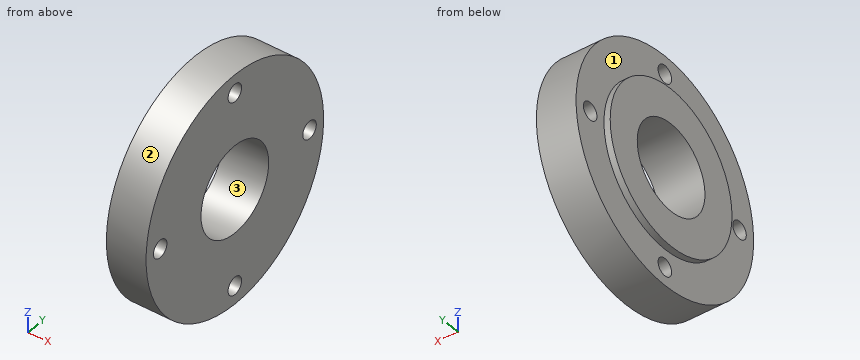
```python
from build123d import *

# Parameters (mm, degrees)
SKETCH1_R             = 32.766
BOSS_EXTRUDE1_DEPTH   = 11.303
SKETCH2_R             = 22.479
BOSS_EXTRUDE2_DEPTH   = 1.778
SKETCH3_R             = 12.5
CUT_EXTRUDE1_DEPTH    = 49.149081746
M6_TAPPED_HOLE1_D     = 5
M6_TAPPED_HOLE1_DEPTH = 12.446
M6_TAPPED_HOLE1_TIP   = 1.502151548


with BuildPart() as part:
    # Sketch1 → Boss-Extrude1 (new body)
    with BuildSketch(Plane(origin=(0, 0, 0), x_dir=(0, 0, -1), z_dir=(1, 0, 0))):
        Circle(SKETCH1_R)
    extrude(amount=-BOSS_EXTRUDE1_DEPTH)

    # Sketch2 → Boss-Extrude2 (add)
    with BuildSketch(Plane.ZY.offset(11.303)):
        with Locations(Location((0, 0, 0), (0, 0, 180))):
            Circle(SKETCH2_R)
    extrude(amount=BOSS_EXTRUDE2_DEPTH)

    # Sketch3 → Cut-Extrude1 (cut, through all)
    with BuildSketch(Plane.ZY.offset(13.081)):
        Circle(SKETCH3_R)
    extrude(amount=-CUT_EXTRUDE1_DEPTH, mode=Mode.SUBTRACT)

    # M6 Tapped Hole1
    with Locations(Plane.ZY.offset(11.303)):
        with Locations((0, 27.559), (27.559, 0), (0, -27.559), (-27.559, 0)):
            Hole(M6_TAPPED_HOLE1_D / 2, depth=M6_TAPPED_HOLE1_DEPTH)
            with Locations((0, 0, -(M6_TAPPED_HOLE1_DEPTH + M6_TAPPED_HOLE1_TIP / 2))):  # 118° drill point
                Cone(0, M6_TAPPED_HOLE1_D / 2, M6_TAPPED_HOLE1_TIP, mode=Mode.SUBTRACT)


solid = part.part
```
For this review, take the finished solid that the model builds, in its own axes (mm). Face numbers are marked on the shaded views. Coordinates: 2 decimals unless noted, no trailing zeros. Loops run counter-clockwise (first coordinate to the right, second up) from the corner with the lowest first, then second, coordinate; pieces in that order, holes last.
1. For line 1 (Y direction, x = -5.25, z = 0); line 2 (Y direction, x = -12.5, z = 0.5); line 3 (Y direction, x = -7.25, z = 1.5), list the stretches that pass through material, from the lowest coordinate up.
2. Insertion check: P1, Ø2, axis at x = -9.5, z = 16, coming from the -Y side; P2, Ø1, axis at x = -10, z = 4, coming from the -Y side; P3, Ø12, axis at y = -14.5, z = 25.5, coming from the -X side; P4, Ø12, axis at y = 5.5, z = 15.5, coming from the +X side. Each pin has a flat end and moves straight along its axis. Give the tip position at first contact, or say it passes through.
3. Add section A-A, the plane y = 0. Give the boundary of the cut face in (x, z), then the cut area to 3 significant figures.
4. Mouldability with a two-part tool opening along Z and no side actions: class the marked faces 1, 2 and 3 as +Z half, -Z half, draft (parallel to the pull), parting line (faces both ways), or undercut.
5. Add section C-C, the plane y = -7.5. Give the boundary of the cut face in (x, z), then the cut area to 3 significant figures.
6. Add section D-D, the plane z = -28.5. Give the boundary of the cut face in (x, y), then the cut area to 3 significant figures.
Result:
1. line 1: y = -32.77 to -30.06, -25.06 to -12.5, 12.5 to 25.06, 30.06 to 32.77
1. line 2: y = -22.47 to -12.49, 12.49 to 22.47
1. line 3: y = -32.73 to -29.56, -25.56 to -12.41, 12.41 to 25.56, 29.56 to 32.73
2. P1: stops at y = -29.13
2. P2: stops at y = -32.58
2. P3: stops at x = -11.3
2. P4: stops at x = 0
3. outline: (-13.08, -22.48) - (-11.3, -22.48) - (-11.3, -25.06) - (0, -25.06) - (0, -12.5) - (-13.08, -12.5) - close; (-13.08, 12.5) - (0, 12.5) - (0, 25.06) - (-11.3, 25.06) - (-11.3, 22.48) - (-13.08, 22.48) - close; (-11.3, -32.77) - (0, -32.77) - (0, -30.06) - (-11.3, -30.06) - close; (-11.3, 30.06) - (0, 30.06) - (0, 32.77) - (-11.3, 32.77) - close
3. area: 381 mm2
4. face 1: draft
4. face 2: parting line
4. face 3: undercut
5. outline: (-13.08, -21.19) - (-11.3, -21.19) - (-11.3, -31.9) - (0, -31.9) - (0, -10) - (-13.08, -10) - close; (-13.08, 10) - (0, 10) - (0, 31.9) - (-11.3, 31.9) - (-11.3, 21.19) - (-13.08, 21.19) - close
5. area: 535 mm2
6. outline: (-11.3, -16.17) - (0, -16.17) - (0, -2.32) - (-11.3, -2.32) - close; (-11.3, 2.32) - (0, 2.32) - (0, 16.17) - (-11.3, 16.17) - close
6. area: 313 mm2
